Check sheet for the modelled part. Datum: model origin and axes. Units: mm. A direction names the side the tool comes from. Give positions to 0.01 mm unless a question says otherwise; leave off trailing zeros. Order: outer loops, then holes, each group sorted by start corner. A loop starts at its lowest first (then second) coordinate and runs counter-clockwise, first axis right, second up.
from build123d import *

# Parameters (mm, degrees)
BOSS_EXTRUDE1_DEPTH = 10
CUT_EXTRUDE1_REACH  = 70.061
SKETCH2_R           = 3
FILLET1_R           = 20
FILLET2_R           = 5
SKETCH3_W           = 29.852045942
SKETCH3_H           = 84.66747525
CUT_EXTRUDE2_DEPTH  = 125


with BuildPart() as part:
    # Sketch1 → Boss-Extrude1 (new body)
    with BuildSketch(Plane.XY):
        with BuildLine():
            Line((13, -5.3170836), (13, -7.9544418))
            Line((13, -7.9544418), (18, -7.9544418))
            Line((18, -7.9544418), (18, 18))
            Line((18, 18), (-8, 18))
            Line((-8, 18), (-8, 36.4526666))
            Line((-8, 36.4526666), (-38.6, 36.4526666))
            Line((-38.6, 36.4526666), (-38.6, -6.6473334))
            Line((-38.6, -6.6473334), (-18, -6.6473334))
            Line((-18, -6.6473334), (-14.542097223, -6.6473334))
            Line((-14.542097223, -6.6473334), (-14.542097223, -1.8473334))
            Line((-14.542097223, -1.8473334), (-33.6, -1.8473334))
            Line((-33.6, -1.8473334), (-33.6, 31.4526666))
            Line((-33.6, 31.4526666), (-12.9, 31.4526666))
            Line((-12.9, 31.4526666), (-12.9, 13))
            Line((-12.9, 13), (-4.305880552, 13))
            Line((-4.305880552, 13), (-4.287512407, 13))
            ThreePointArc((-4.287512407, 13), (-3.333616586, 12.604883414), (-2.9385, 11.650987593))
            Line((-2.9385, 11.650987593), (-2.9385, 11.539212407))
            ThreePointArc((-2.9385, 11.539212407), (-3.333616586, 10.585316586), (-4.287512407, 10.1902))
            Line((-4.287512407, 10.1902), (-6.476788598, 10.1902))
            ThreePointArc((-6.476788598, 10.1902), (-7.154992901, 9.736757749), (-6.995146796, 8.93674514))
            Line((-6.995146796, 8.93674514), (-3.686383353, 5.635543623))
            ThreePointArc((-3.686383353, 5.635543623), (-2.754473742, 5.014017446), (-1.655778399, 4.7958))
            Line((-1.655778399, 4.7958), (1.655778399, 4.7958))
            ThreePointArc((1.655778399, 4.7958), (2.754473742, 5.014017446), (3.686383353, 5.635543623))
            Line((3.686383353, 5.635543623), (6.995146796, 8.93674514))
            ThreePointArc((6.995146796, 8.93674514), (7.154992901, 9.736757749), (6.476788598, 10.1902))
            Line((6.476788598, 10.1902), (4.287512407, 10.1902))
            ThreePointArc((4.287512407, 10.1902), (3.333616586, 10.585316586), (2.9385, 11.539212407))
            Line((2.9385, 11.539212407), (2.9385, 11.650987593))
            ThreePointArc((2.9385, 11.650987593), (3.333616586, 12.604883414), (4.287512407, 13))
            Line((4.287512407, 13), (5.321597603, 13))
            Line((5.321597603, 13), (10.5918, 13))
            ThreePointArc((10.5918, 13), (12.29465455, 12.29465455), (13, 10.5918))
            Line((13, 10.5918), (13, 7.9544418))
            Line((13, 7.9544418), (13, 5.3170836))
            Line((13, 5.3170836), (13, 4.287469289))
            ThreePointArc((13, 4.287469289), (12.604883414, 3.333573468), (11.650987593, 2.938456882))
            Line((11.650987593, 2.938456882), (11.539212407, 2.938456882))
            ThreePointArc((11.539212407, 2.938456882), (10.585316586, 3.333573468), (10.1902, 4.287469289))
            Line((10.1902, 4.287469289), (10.1902, 6.402089023))
            ThreePointArc((10.1902, 6.402089023), (9.74154152, 7.073969797), (8.94902056, 6.917034355))
            Line((8.94902056, 6.917034355), (5.652895046, 3.628441884))
            ThreePointArc((5.652895046, 3.628441884), (5.027976112, 2.694919539), (4.8085, 1.593185507))
            Line((4.8085, 1.593185507), (4.8085, -1.593185507))
            ThreePointArc((4.8085, -1.593185507), (5.027976112, -2.694919539), (5.652895046, -3.628441884))
            Line((5.652895046, -3.628441884), (8.94902056, -6.917034355))
            ThreePointArc((8.94902056, -6.917034355), (9.74154152, -7.073969797), (10.1902, -6.402089023))
            Line((10.1902, -6.402089023), (10.1902, -4.287469289))
            ThreePointArc((10.1902, -4.287469289), (10.585316586, -3.333573468), (11.539212407, -2.938456882))
            Line((11.539212407, -2.938456882), (11.650987593, -2.938456882))
            ThreePointArc((11.650987593, -2.938456882), (12.604883414, -3.333573468), (13, -4.287469289))
            Line((13, -4.287469289), (13, -5.3170836))
        make_face()
    extrude(amount=BOSS_EXTRUDE1_DEPTH)

    # Sketch2 → Cut-Extrude1 (cut, up to next)
    with BuildSketch(Plane.ZY.offset(38.6), mode=Mode.PRIVATE) as cut_extrude1_sk1:
        with Locations((4.5, 26.4526666)):
            Circle(SKETCH2_R)
    cut_extrude1_tool1 = extrude(cut_extrude1_sk1.sketch, amount=-CUT_EXTRUDE1_REACH, mode=Mode.PRIVATE) & part.part
    # Sketch2 → Cut-Extrude1 (cut, up to next)
    with BuildSketch(Plane.ZY.offset(38.6), mode=Mode.PRIVATE) as cut_extrude1_sk2:
        with Locations((4.5, 7.9526666)):
            Circle(SKETCH2_R)
    cut_extrude1_tool2 = extrude(cut_extrude1_sk2.sketch, amount=-CUT_EXTRUDE1_REACH, mode=Mode.PRIVATE) & part.part
    add(cut_extrude1_tool1.solids().sort_by_distance((-38.6, 26.452667, 4.5))[0], mode=Mode.SUBTRACT)
    add(cut_extrude1_tool2.solids().sort_by_distance((-38.6, 7.952667, 4.5))[0], mode=Mode.SUBTRACT)

    # Fillet1
    # the kernel refuses this fillet: 20 mm, written as the material it adds along each edge
    with BuildSketch(Plane(origin=(-8, 18, 0), x_dir=(1, 0, 0), z_dir=(0, 0, 1))) as fillet1_piece_1:
        with BuildLine():
            CenterArc((19.940054146, 20), FILLET1_R, 184.437217766, 85.562782234)
            Line((0, 18.4526666), (-0.398801083, 18.421719932))
            ThreePointArc((-0.398801083, 18.421719932), (-0.4, 9.2263333), (-0.4, 0))
            Line((-0.4, 0), (0, -0.4))
            Line((0, -0.4), (19.940054146, -0.4))
            Line((19.940054146, -0.4), (19.940054146, 0))
        make_face()
    extrude(amount=10)

    # Fillet2
    fillet2_edges = [part.edges().sort_by_distance(p)[0] for p in [
        (-38.6, -6.6473334, 5),
        (-38.6, 36.4526666, 5),
        (18, 18, 5),
    ]]
    fillet(fillet2_edges, radius=FILLET2_R)


with BuildPart() as body_2:
    # Mirror1: mirrored copy
    add(part.part.mirror(Plane.XY))


with BuildPart() as part_1:
    add(part.part)

    # Sketch3 → Cut-Extrude2 (cut)
    with BuildSketch(Plane.ZY.offset(38.6)):
        with Locations((14.926022971, 7.66612184)):
            Rectangle(SKETCH3_W, SKETCH3_H)
    extrude(amount=-CUT_EXTRUDE2_DEPTH, mode=Mode.SUBTRACT)


solid = body_2.part
1) Set-up check for faces 3 (the face through (7.324, 5.296, -4.93)), 4 (the face through (-36.135, 23.524, -3.85)), 5 (the face through (10.19, -5, -5)): record each of +Z, -Z, +X, -X, +Y, -Y from which the full face is reachable in a straight line by a thin tool's end or side.
Recorded:
face 3: +Z, -Z
face 4: -X
face 5: +Z, -Z, -Y
2) Draft check along X on faces 1 (the face through (-10, 15, -10)), 2 (the face through (13, 7, -5)). Enter one of: +X half, -X half, draft (parallel to the pull), parting line (faces both ways), or undercut.
Recorded:
face 1: draft
face 2: undercut
3) Section check A-A, the plane x = -27. Record the cut outline in (y, z).
Recorded:
outline: (-6.65, -10) - (-1.85, -10) - (-1.85, 0) - (-6.65, 0) - close; (31.45, -10) - (36.45, -10) - (36.45, 0) - (31.45, 0) - close
4) Material ranges on L1, parallel to Y at x = -20.5, z = -6; L2, parallel to X at y = 12, z = -7.25; L3, parallel to X at y = 4, z = -3.5, recorded low to high.
Recorded:
L1: y = -6.65 to -1.85, 31.45 to 36.45
L2: x = -38.6 to -33.6, -2.98 to 2.98, 12.55 to 18
L3: x = -38.6 to -33.6, 6.03 to 10.22, 12.97 to 18
5) Section check B-B, the plane z = -4.5. State how many separate pieces and enclosed holes the cut face has, then the cut area to 3 significant figures.
Recorded:
separate pieces: 3
enclosed holes: 0
area: 922 mm2
6) Section check C-C, the plane y = 34. Record the cut outline in (x, z).
Recorded:
outline: (-37.9, -10) - (-7.66, -10) - (-7.66, 0) - (-37.9, 0) - close
7) Depth check by flat-ended pin: pin 1 Ø1 at (x, z) = (7, -6) entering from +Y; pin 2 Ø4.5 at (x, z) = (-9, -6.5) entering from -Y; pin 3 Ø3.5 at (y, z) = (26.45, -4.5) entering from -X; pin 4 Ø6 at (x, y) = (-0.5, 1.5) entering from -Z. Enter the tip coordinate at first touch or a pass-through.
Recorded:
pin 1: stops at y = 18.75
pin 2: stops at y = 8.69
pin 3: stops at x = -12.9
pin 4: passes through
